Could you check a few things on this drawing? It's one solid part, dimensions in mm from its lowest x, y, z. Give positions to 0.01 mm unless a question says otherwise; leave off trailing zeros. Order: outer loops, then holes, each group sorted by start corner. A loop starts at its lowest first (then second) coordinate and runs counter-clockwise, first axis right, second up. Notation, with made-up numbers: M -30,59.5 L -12,59.5 A29 ccw -12,80.5 Z; hole C -27.5,41 d2. An arc over 180 degrees is marked long. Use one line per item in the form item = value. Start each with the question number.
1. I want a section at A-A, the plane y = 38. List the corners of the cut face in (x, z) for me, and give its area (3 significant figures).
2. I want a section at B-B, the plane x = 3.25. List the corners of the cut face in (y, z) for me (1 decimal).
3. I want a section at C-C, the plane z = 0.7. Count the separate pieces of the cut face and the enclosed holes in it, and give its area (3 significant figures).
4. Will this pin go through, and if not, where does the flat tip stop? P1, Ø2, axis at x = 12.25, y = 78, coming from the -Z side.
5. I need wall thicknesses on L1, parallel to X at y = 78, z = 1.9; L2, parallel to Y at x = 12.75, z = 1.15 (1 decimal); L3, parallel to Y at x = 16, z = 1.9 (1 decimal). Which ranges of each line are inside material? Lowest first, please.
6. I want a section at D-D, the plane y = 49. List the corners of the cut face in (x, z) for me.
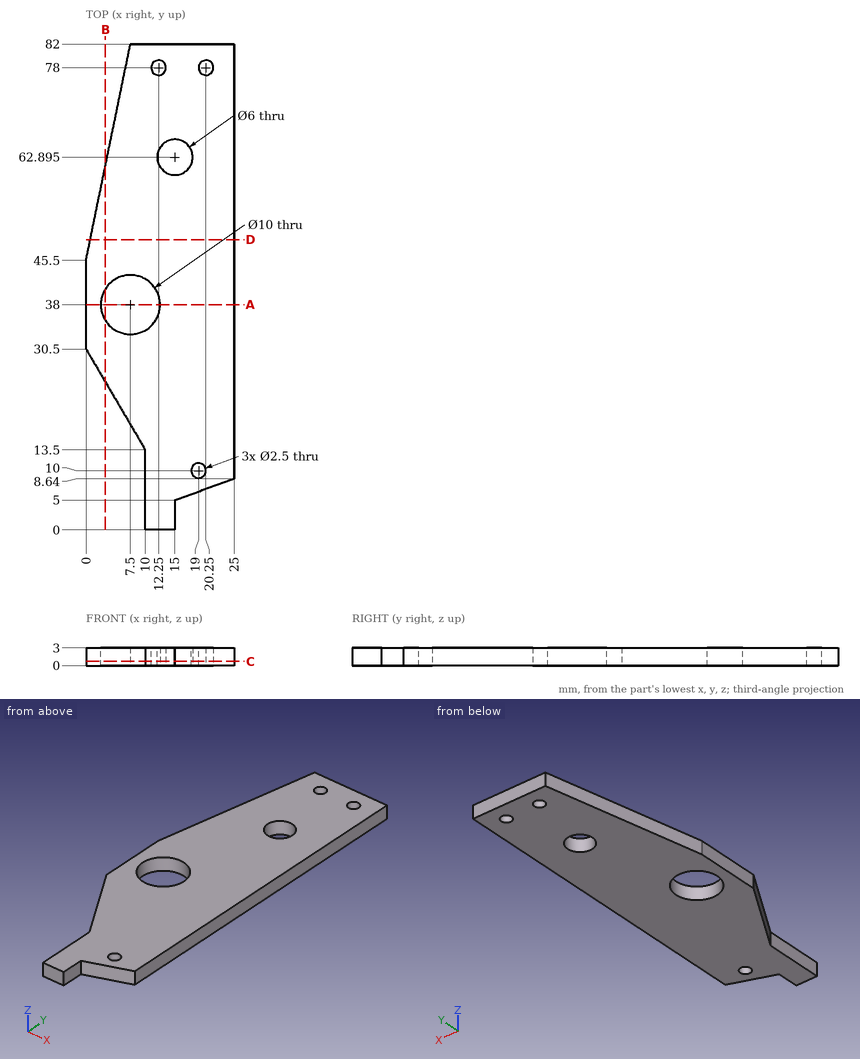
Check result:
q1.outline = M 0,0 L 2.5,0 L 2.5,3 L 0,3 Z; M 12.5,0 L 25,0 L 25,3 L 12.5,3 Z
q1.area = 45.0 mm2
q2.outline = M 25,0 L 35.4,0 L 35.4,3 L 25,3 Z; M 40.6,0 L 61.3,0 L 61.3,3 L 40.6,3 Z
q3.separate_pieces = 1
q3.enclosed_holes = 5
q3.area = 1,500 mm2
q4.P1 = through
q5.L1 = 6.68 to 11, 13.5 to 19, 21.5 to 25
q5.L2 = 0 to 60.9, 64.9 to 76.9, 79.1 to 82
q5.L3 = 5.4 to 60.1, 65.7 to 82
q6.outline = M 0.72,0 L 25,0 L 25,3 L 0.72,3 Z
